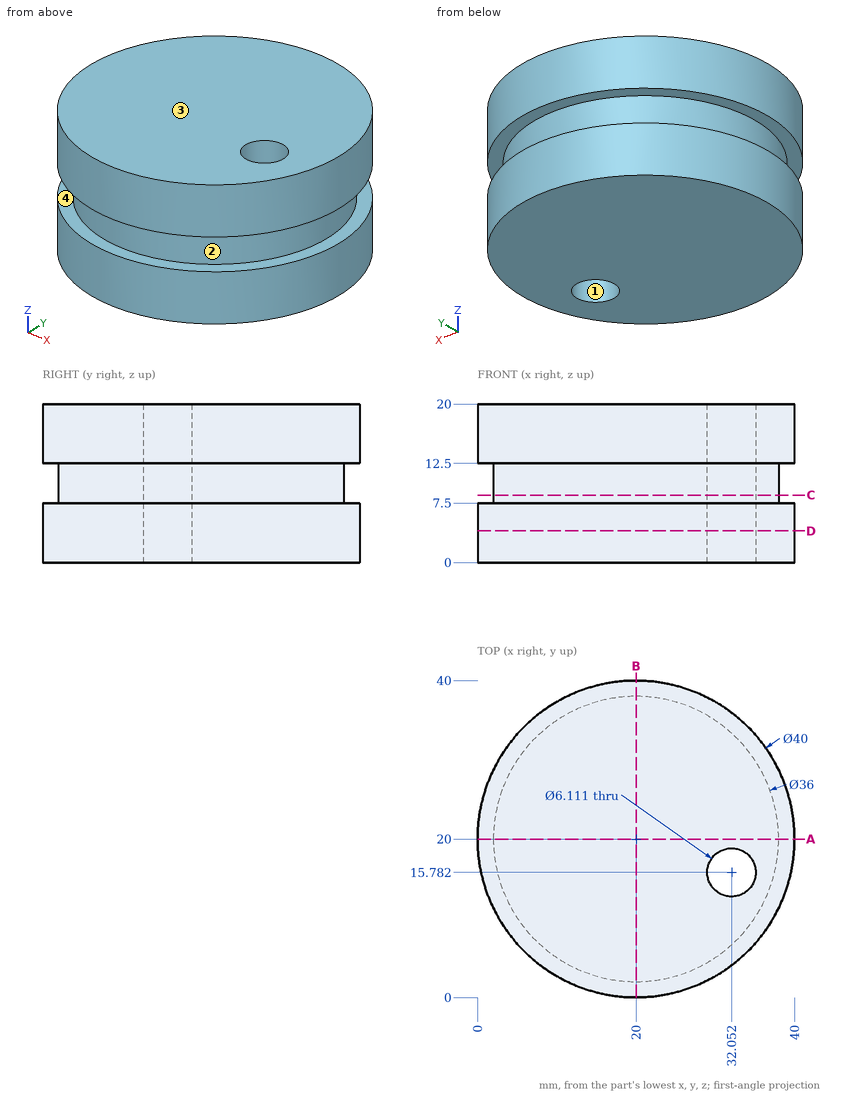
Study the drawing (mm; zero at the part's minimum x, y, z) and answer. Coordinates: 2 decimals unless noted, no trailing zeros. Order: outer loops, then holes, each group sorted by start corner. A loop starts at its lowest first (then second) coordinate and runs counter-clockwise, first axis right, second up. Notation, with made-up numbers: (59.5, 19.25) -> (98.5, 19.25) arc R20 ccw to (98.5, 55.25) -> close; hole circle Ø9 at (14, 41.5). An arc over 180 degrees is marked (long way). Answer in a Markdown table with one row per item. Add a question column.
Item 1: Find the intervals of material crossed by L1, parallel to Z at x = 28, y = 37; L2, parallel to X at y = 15.5, z = 8 (1 decimal); L3, parallel to Y at x = 25.5, z = 10.25, in increasing order. Write a range as from..to.
Item 2: Find section D-D (z = 4). Write down the section's boundary in (x, y) (1 decimal), then the cut area to 3 significant figures.
Item 3: Determine the mould class of the marked faces 1, 2, 3 and 4 for opening direction Z: +Z half, -Z half, draft (parallel to the pull), parting line (faces both ways), or undercut.
Item 4: Find section A-A (y = 20). Write down the section's boundary in (x, z).
Item 5: Find section C-C (z = 8.5). Write down the section's boundary in (x, y) (1 decimal).
Item 6: Each of these flat-tipped pins is pushed along its axis until it touches: P1, Ø10, axis at x = 28.5, z = 2.5, coming from the +Y side; P2, Ø3, axis at x = 33.5, z = 10.5, coming from the -Y side (1 decimal); P3, Ø4, axis at x = 12, z = 15.5, coming from the +Y side; P4, Ø10, axis at y = 20.5, z = 3, coming from the -X side. Where does it stop, or does it pass through?
Result set:
| question | item | result |
|---|---|---|
| 1 | L1 | z = 0..7.5, 12.5..20 |
| 1 | L2 | x = 2.6..29, 35.1..37.4 |
| 1 | L3 | y = 2.86..37.14 |
| 2 | outline | circle Ø40 at (20, 20); hole circle Ø6.1 at (32.1, 15.8) |
| 2 | area | 1,230 mm² |
| 3 | face 1 | draft |
| 3 | face 2 | undercut |
| 3 | face 3 | +Z half |
| 3 | face 4 | undercut |
| 4 | outline | (0, 0) -> (40, 0) -> (40, 7.5) -> (38, 7.5) -> (38, 12.5) -> (40, 12.5) -> (40, 20) -> (0, 20) -> (0, 12.5) -> (2, 12.5) -> (2, 7.5) -> (0, 7.5) -> close |
| 5 | outline | circle Ø36 at (20, 20); hole circle Ø6.1 at (32.1, 15.8) |
| 6 | P1 | stops at y = 39.69 |
| 6 | P2 | stops at y = 6.6 |
| 6 | P3 | stops at y = 39.08 |
| 6 | P4 | stops at x = 0 |
